Design review of the part built by this model. Coordinates are the model's own, in mm. Face numbers are marked on the shaded views. Coordinates: 2 decimals unless noted, no trailing zeros. Write each loop counter-clockwise with the first axis right and the second up, starting at its lowest first coordinate (ties: lowest second). Pieces come first, ordered by that corner, then holes.
Q1. Take a section at C-C (x = -7). Give the boundary of the cut face in (y, z), and give its area (3 significant figures).
Q2. Insertion check: pin 1 (6 mm diameter, centred on y = 10.5, z = -3, fed in from +X). The pin has a flat end and moves straight along its axis. Give the tip position at first contact, or say it passes through.
Q3. Take a section at B-B (y = 8). Give the boundary of the cut face in (x, z).
Q4. Mouldability with a two-part tool opening along Y and no side actions: class the marked faces 1, 2, 3 and 4 as pulls with the +Y half, pulls with the -Y half, needs draft (parallel to the pull), parting line crosses it, or undercut.
Q5. Take a section at D-D (z = -7). Give the boundary of the cut face in (x, y).
Q6. For probe 1 along Y at (x, z) = (-6.25, 12); probe 2 along X at (y, z) = (17.75, -7.5); probe 3 along Z at (x, y) = (-6.75, 4.75), list the stretches that pass through material, from the lowest coordinate up.
Q7. Take a section at A-A (z = 12). Give the boundary of the cut face in (x, y).
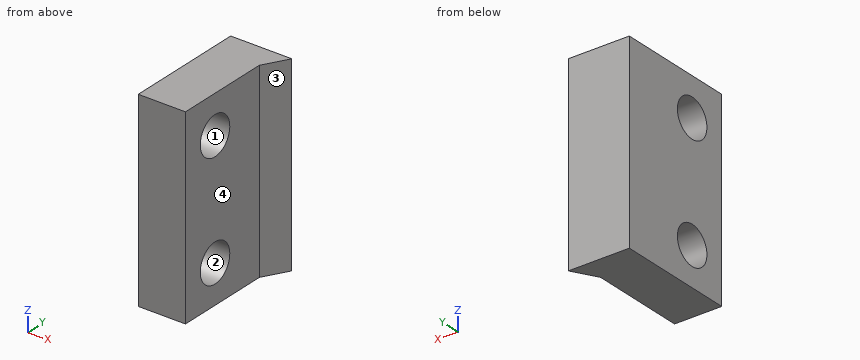
```python
from build123d import *

# Parameters (mm, degrees)
BOSS_EXTRUDE1_DEPTH = 20
SKETCH4_R           = 3.99415
CUT_EXTRUDE1_DEPTH  = 13.7


with BuildPart() as part:
    # Sketch2 → Boss-Extrude1 (new body, symmetric)
    with BuildSketch(Plane.XY):
        Polygon((0, 0), (-9.813248654, 0), (-9.813248654, 25), (2.886751346, 25), (0, 20), align=None)
    extrude(amount=BOSS_EXTRUDE1_DEPTH, both=True)

    # Sketch4 → Cut-Extrude1 (cut, through all)
    with BuildSketch(Plane.ZY.offset(9.813248654)):
        with Locations((-12, 8)):
            Circle(SKETCH4_R)
    cut_extrude1 = extrude(amount=-CUT_EXTRUDE1_DEPTH, mode=Mode.SUBTRACT)

    # Mirror1: Cut-Extrude1 across plane
    add(cut_extrude1.mirror(Plane.XY), mode=Mode.SUBTRACT)


solid = part.part
```
Response:
1. outline: (0, -20) - (25, -20) - (25, 20) - (0, 20) - close; hole circle Ø7.99 at (8, -12); hole circle Ø7.99 at (8, 12)
1. area: 900 mm2
2. pin 1: stops at x = 0
3. outline: (-9.81, -20) - (0, -20) - (0, -15.99) - (-9.81, -15.99) - close; (-9.81, -8.01) - (0, -8.01) - (0, 8.01) - (-9.81, 8.01) - close; (-9.81, 15.99) - (0, 15.99) - (0, 20) - (-9.81, 20) - close
4. face 1: undercut
4. face 2: undercut
4. face 3: pulls with the -Y half
4. face 4: needs draft
5. outline: (-9.81, 0) - (0, 0) - (0, 20) - (2.89, 25) - (-9.81, 25) - close
6. probe 1: y = 0 to 4.01, 11.99 to 25
6. probe 2: x = -9.81 to 0
6. probe 3: z = -20 to -14.32, -9.68 to 9.68, 14.32 to 20
7. outline: (-9.81, 0) - (0, 0) - (0, 4.01) - (-9.81, 4.01) - close; (-9.81, 11.99) - (0, 11.99) - (0, 20) - (2.89, 25) - (-9.81, 25) - close
